Here's how the part is built. I have some questions about the finished solid (model axes, mm). A direction names the side the tool comes from. Coordinates: 2 decimals unless noted, no trailing zeros. Write each loop counter-clockwise with the first axis right and the second up, starting at its lowest first coordinate (ties: lowest second). Pieces come first, ordered by that corner, then holes.
Item 1: For faces 1 (the face through (60, 25, 2)), 2 (the face through (4, 39, 8)), 3 (the face through (32, 45, -2)), 4 (the face through (16.5, 35, 42)), which set-ups out of +Z, -Z, +X, -X, +Y, -Y let a thin tool reach every point of the face, with its end or its side?
Item 2: I'm going to push flat-ended pins straight in: P1, Ø0.8, axis at x = 47.5, y = 35.5, coming from the -Z side; P2, Ø1, axis at x = 37, y = 34, coming from the -Z side; P3, Ø4, axis at x = 9.5, z = 35, coming from the -Y side; P4, Ø3, axis at x = 12, z = 18, coming from the -Y side. Where does each tip first touch, or does it pass through?
Item 3: If we mould it in two halves opening along Z, with no side actions, what happens to faces 5 (the face through (46.75, 35, 40)), 6 (the face through (1.972, 37.395, 8.916)), 7 (the face through (25.265, 47.028, 8.228)), 8 (the face through (19, 25, 41))? For each: pulls with the +Z half, pulls with the -Z half, needs draft (parallel to the pull), parting line crosses it, or undercut.
Item 4: I want a section at D-D (x = 30). Please give me the cut outline in (y, z).
Item 5: I want a section at B-B (z = 23.5). Please give me the cut outline in (x, y), and give its area (3 significant figures).
Item 6: Please list where these lines run through material, in increasing order: line 1 (Z direction, x = 40, y = 47); line 2 (Z direction, x = 12, y = 47.05); line 3 (X direction, y = 47, z = 33).
Item 7: I want a section at C-C (x = 40). Please give me the cut outline in (y, z), and give its area (3 significant figures).
Item 8: I want a section at A-A (y = 12). Please give me the cut outline in (x, z).
Autodesk Inventor part; units mm, degrees
ref_plane "Work Plane1" through (20, 2, 0) normal (-1, 0, 0) x (0, 0, 1)
ref_plane "YZ Plane" through (0, 0, 0) normal (1, 0, 0) x (0, 1, 0)
ref_plane "XZ Plane" through (0, 0, 0) normal (0, 1, 0) x (-1, 0, 0)
sketch "Sketch1" plane through (0, 0, 0) normal (0, 0, 1) x (1, 0, 0)
  line L0 (0, 0) -> (64, 0)
  line L1 (64, 0) -> (64, 45)
  line L2 (64, 45) -> (0, 45)
  line L3 (0, 45) -> (0, 0)
  circle A0 centre (12, 33) radius 6
  circle A1 centre (52, 33) radius 6
  circle A2 centre (30, 31) radius 1.75
  circle A3 centre (13, 12) radius 1.75
  dimension "d0" = 64
  dimension "d1" = 45
  dimension "d2" = 12
  dimension "d3" = 12
  dimension "d4" = 12
  dimension "d5" = 12
  dimension "d6" = 3.5
  dimension "d7" = 30
  dimension "d8" = 14
  dimension "d9" = 3.5
  dimension "d10" = 13
  dimension "d11" = 33
extrude "Extrusion1" add sketch "Sketch1" along normal blind 3
sketch "Sketch2" plane through (0, 0, 3) normal (0, 0, 1) x (1, 0, 0)
  line L0 (0, 0) -> (64, 0)
  line L1 (64, 0) -> (34, 0)
  line L2 (34, 0) -> (34, 25)
  line L3 (34, 25) -> (64, 25)
  line L4 (64, 25) -> (64, 0)
  dimension "d14" = 30
  dimension "d15" = 25
extrude "Extrusion2" cut sketch "Sketch2" against normal blind 3
fillet "Fillet1" radius 2 4 edges at (34, 25, 1.5) (64, 25, 1.5) (34, 0, 1.5) (0, 0, 1.5)
sketch "Sketch5" plane through (0, 45, 0) normal (0, 1, 0) x (1, 0, 0)
  line L0 (64, -3) -> (0, -3)
  line L1 (0, -3) -> (64, -3)
  line L2 (64, -3) -> (64, 8)
  line L3 (64, 8) -> (0, 8)
  line L4 (0, 8) -> (0, -3)
  point P0 (0, 0)
  dimension "d20" = 11
  dimension "d21" = 64
extrude "Extrusion3" add sketch "Sketch5" along normal blind 4
sketch "Sketch6" plane through (0, 0, 3) normal (0, 0, 1) x (1, 0, 0)
  line L0 (0, 49) -> (64, 49)
  line L1 (64, 27) -> (64, 49)
  line L2 (0, 49) -> (64, 49)
  line L3 (64, 49) -> (64, 45)
  line L4 (64, 45) -> (0, 45)
  line L5 (0, 45) -> (0, 49)
  point P0 (0, 0)
  dimension "d24" = 4
extrude "Extrusion4" add sketch "Sketch6" along normal blind 40
sketch "Sketch7" plane through (0, 45, 3) normal (0, -1, 0) x (1, 0, 0)
  line L0 (61, 20) -> (35, 20)
  line L1 (35, 20) -> (35, 0)
  line L2 (35, 0) -> (61, 0)
  line L3 (61, 0) -> (61, 20)
  line L4 (0, 40) -> (64, 40)
  line L5 (64, 0) -> (64, 40)
  point P0 (0, -3)
  dimension "d27" = 20
  dimension "d28" = 3
  dimension "d29" = 20
  dimension "d30" = 26
extrude "Extrusion5" cut sketch "Sketch7" against normal blind 40
sketch "Sketch8" plane through (0, 45, 43) normal (0, -1, 0) x (1, 0, 0)
  line L0 (35, -20) -> (61, -20)
  line L1 (61, -20) -> (61, -40)
  line L2 (35, -40) -> (35, -20)
  line L3 (35, -40) -> (0, -40)
  point P0 (0, -43)
  point P1 (56, -10)
  point P2 (40, -10)
  point P3 (27, -25)
  point P4 (27, -35)
  point P5 (12, -35)
  point P6 (12, -25)
  point P7 (12, -10)
  point P8 (27, -10)
  dimension "d33" = 10
  dimension "d34" = 10
  dimension "d35" = 5
  dimension "d36" = 5
  dimension "d37" = 5
  dimension "d38" = 8
  dimension "d39" = 8
  dimension "d40" = 5
  dimension "d63" = 15
hole "Hole1" at (56, 45, 33) at (40, 45, 33) at (27, 45, 18) at (27, 45, 8) at (12, 45, 8) at (12, 45, 18) at (12, 45, 33) at (27, 45, 33) direction (0, 1, 0) diameter 3.5 end through all
sketch "Sketch10" plane through (0, 2, 0) normal (-1, 0, 0) x (0, 0, 1)
  line L0 (3, 28) -> (15, 43)
  line L1 (3, 43) -> (43, 43)
  line L2 (3, 43) -> (3, 28)
  line L3 (3, 37) -> (3, 25)
  line L4 (3, 43) -> (15, 43)
  point P0 (0, -2)
  dimension "d48" = 15
  dimension "d49" = 12
extrude "Extrusion6" add sketch "Sketch10" against normal blind 4
sketch "Sketch11" plane through (64, 27, 3) normal (1, 0, 0) x (0, 0, -1)
  line L0 (0, 0) -> (0, 12)
  line L1 (0, 3) -> (0, 18)
  line L2 (0, 18) -> (-12, 18)
  line L3 (0, 18) -> (-20, 18)
  line L4 (0, 3) -> (-12, 18)
  point P0 (3, -27)
  dimension "d52" = 12
  dimension "d53" = 15
extrude "Extrusion7" add sketch "Sketch11" against normal blind 3
ref_plane "Work Plane1" through (20, 2, 0) normal (-1, 0, 0) x (0, 0, 1)
sketch "Sketch12" plane through (20, 2, 0) normal (-1, 0, 0) x (0, 0, 1)
  line L0 (3, 43) -> (3, 28)
  line L1 (3, 43) -> (3, 28)
  line L2 (15, 43) -> (3, 28)
  line L3 (3, 28) -> (15, 43)
  line L4 (15, 43) -> (3, 43)
  point P0 (0, -2)
extrude "Extrusion8" add sketch "Sketch12" along normal mid plane 3
sketch "Sketch13" plane through (0, 45, 0) normal (0, -1, 0) x (1, 0, 0)
  line L0 (0, -8) -> (0, 0)
  line L1 (64, -8) -> (64, 43)
  line L2 (0, -8) -> (64, -8)
  line L3 (64, -8) -> (64, -3)
  line L4 (64, -3) -> (0, -3)
  line L5 (0, -3) -> (0, -8)
  dimension "d59" = 5
extrude "Extrusion9" add sketch "Sketch13" along normal blind 5
sketch "Sketch14" plane through (0, 45, 43) normal (0, -1, 0) x (1, 0, 0)
  line L0 (64, 0) -> (0, 0)
  line L1 (16.5, 0) -> (22.5, 0)
  line L2 (22.5, -2) -> (22.5, 0)
  line L3 (22.5, -2) -> (20.75, -2)
  line L4 (20.75, -2) -> (20.75, -4)
  line L5 (20.75, -4) -> (18.25, -4)
  line L6 (18.25, -4) -> (18.25, -2)
  line L7 (18.25, -2) -> (16.5, -2)
  line L8 (16.5, -2) -> (16.5, 0)
  line L9 (45, 0) -> (45, -2)
  line L10 (45, -2) -> (46.75, -2)
  line L11 (46.75, -2) -> (46.75, -4)
  line L12 (46.75, -4) -> (49.25, -4)
  line L13 (49.25, -4) -> (49.25, -2)
  line L14 (49.25, -2) -> (51, -2)
  line L15 (51, -2) -> (51, 0)
  line L16 (45, 0) -> (51, 0)
  point P0 (0, -43)
  dimension "d64" = 2
  dimension "d65" = 2.5
  dimension "d66" = 6
  dimension "d67" = 2.5
  dimension "d68" = 6
  dimension "d70" = 2
  dimension "d72" = 16.5
  dimension "d73" = 13
extrude "Extrusion10" add sketch "Sketch14" along normal blind 20
sketch "Sketch16" plane through (0, 49, 0) normal (0, 1, 0) x (1, 0, 0)
  line L0 (35, -23) -> (61, -23)
  line L1 (61, -23) -> (61, -28)
  line L2 (61, -28) -> (35, -28)
  line L3 (35, -28) -> (35, -23)
  point P0 (0, 0)
  dimension "d86" = 26
  dimension "d87" = 5
extrude "Extrusion12" cut sketch "Sketch16" against normal blind 10
sketch "Sketch17" plane through (0, 0, 3) normal (0, 0, 1) x (1, 0, 0)
  circle A0 centre (52, 33) radius 6
  line L0 (62, 25) -> (36, 25)
  line L1 (46, 33) -> (58, 33)
  line L2 (58, 33) -> (58, 25)
  line L3 (58, 25) -> (46, 25)
  line L4 (46, 25) -> (46, 33)
  point P0 (0, 0)
extrude "Extrusion13" cut sketch "Sketch17" against normal blind 10 contours L2 L0 L4 A0 | A0 L1 picked at (51.2908, 31.13)
equation "\"d3\" = d2"
equation "\"d6\" = d9"
equation "\"d67\" = d65"
properties part number "PLACA_BASE"
Answer:
1. face 1: +Z, -Z, +X, -Y
1. face 2: +Z, -Y
1. face 3: +X, -X, -Y
1. face 4: +Z, -X, -Y
2. P1: stops at z = 39
2. P2: stops at z = 0
2. P3: stops at y = 45
2. P4: passes through
3. face 5: undercut
3. face 6: pulls with the +Z half
3. face 7: undercut
3. face 8: needs draft
4. outline: (0, 0) - (29.25, 0) - (29.25, 3) - (0, 3) - close; (32.75, 0) - (45, 0) - (45, -3) - (40, -3) - (40, -8) - (49, -8) - (49, 43) - (45, 43) - (45, 3) - (32.75, 3) - close
5. outline: (0, 45) - (35, 45) - (35, 49) - (0, 49) - close; (61, 45) - (64, 45) - (64, 49) - (61, 49) - close
5. area: 152 mm2
6. line 1: z = -8 to 3, 28 to 31.25, 34.75 to 43
6. line 2: z = -8 to 6.25, 9.75 to 16.25, 19.75 to 31.25, 34.75 to 43
6. line 3: x = 0 to 10.25, 13.75 to 25.25, 28.75 to 38.25, 41.75 to 54.25, 57.75 to 64
7. outline: (25, 0) - (45, 0) - (45, -3) - (40, -3) - (40, -8) - (49, -8) - (49, 3) - (25, 3) - close; (45, 28) - (49, 28) - (49, 31.25) - (45, 31.25) - close; (45, 34.75) - (49, 34.75) - (49, 43) - (45, 43) - close
7. area: 175 mm2
8. outline: (0, 0) - (11.25, 0) - (11.25, 3) - (0, 3) - close; (14.75, 0) - (34, 0) - (34, 3) - (14.75, 3) - close
